Read the model definition and answer for the solid it produces. Units are mm, in the model's axes. A direction names the side the tool comes from. Coordinates: 2 decimals unless noted, no trailing zeros. Loops run counter-clockwise (first coordinate to the right, second up) from the corner with the lowest first, then second, coordinate; pieces in that order, holes last. Notation, with made-up numbers: M 18,-10.5 L 66,-10.5 A19 ccw 66,-0.5 Z; hole C -11.5,-0.5 d8. An arc over 180 degrees is marked long. One line per item, written item: value. Start each with the question number.
```python
from build123d import *

# Parameters (mm, degrees)
SKETCH1_W           = 20.5
SKETCH1_H           = 16.25
SKETCH1_R           = 1.625
BOSS_EXTRUDE1_DEPTH = 1.6
FILLET1_R           = 1
SKETCH2_W           = 2.5
SKETCH2_H           = 8
BOSS_EXTRUDE2_DEPTH = 2.5
FILLET2_R           = 0.5
SKETCH8_W           = 0.55
SKETCH8_H           = 0.55
SKETCH9_W           = 0.55
SKETCH9_H           = 0.55
SKETCH12_W          = 0.55
SKETCH12_H          = 0.55
SKETCH13_W          = 1.45
SKETCH13_H          = 1
CUT_EXTRUDE1_DEPTH  = 4


with BuildPart() as part:
    # Sketch1 → Boss-Extrude1 (new body)
    with BuildSketch(Plane(origin=(0, 0, 0), x_dir=(1, 0, 0), z_dir=(0, 1, 0))):
        Rectangle(SKETCH1_W, SKETCH1_H)
        with Locations(Location((7.625, 5.7, 0), (0, 0, 270))):
            Circle(SKETCH1_R, mode=Mode.SUBTRACT)
        with Locations(Location((7.625, -5.7, 0), (0, 0, 90))):
            Circle(SKETCH1_R, mode=Mode.SUBTRACT)
    extrude(amount=BOSS_EXTRUDE1_DEPTH)

    # Fillet1
    fillet1_edges = [part.edges().sort_by_distance(p)[0] for p in [
        (10.25, 0.8, 8.125),
        (-10.25, 0.8, 8.125),
        (-10.25, 0.8, -8.125),
        (10.25, 0.8, -8.125),
    ]]
    fillet(fillet1_edges, radius=FILLET1_R)

    # Sketch2 → Boss-Extrude2 (add)
    with BuildSketch(Plane(origin=(0, 1.6, 0), x_dir=(1, 0, 0), z_dir=(0, 1, 0))):
        with Locations((-9, 0)):
            Rectangle(SKETCH2_W, SKETCH2_H)
    extrude(amount=BOSS_EXTRUDE2_DEPTH)

    # Fillet2
    fillet2_edges = [part.edges().sort_by_distance(p)[0] for p in [
        (-7.75, 2.85, 4),
        (-7.75, 2.85, -4),
        (-10.25, 2.85, -4),
        (-10.25, 2.85, 4),
    ]]
    fillet(fillet2_edges, radius=FILLET2_R)

    # Sweep2: sweep along a path in Sketch5
    with BuildLine(Plane.XY.offset(-2.5)) as sweep2_path:
        Line((-9, 4.1), (-9, 4.85))
        ThreePointArc((-9, 4.85), (-8.682958383, 5.34027213), (-8.160059174, 5.6))
        Line((-8.160059174, 5.6), (-1, 5.6))
    # Sketch8 → Sweep2 (sweep)
    with BuildSketch(Plane(origin=(0, 4.1, 0), x_dir=(1, 0, 0), z_dir=(0, 1, 0))):
        with Locations((-9.001105099, 2.502876889)):
            Rectangle(SKETCH8_W, SKETCH8_H)
    sweep(path=sweep2_path.line, transition=Transition.RIGHT)

    # Sweep3: sweep along a path in Sketch6
    with BuildLine(Plane.XY.offset(2.5)) as sweep3_path:
        Line((-9, 4.1), (-9, 4.85))
        ThreePointArc((-9, 4.85), (-8.682958383, 5.34027213), (-8.160059174, 5.6))
        Line((-8.160059174, 5.6), (-1, 5.6))
    # Sketch9 → Sweep3 (sweep)
    with BuildSketch(Plane(origin=(0, 4.1, 0), x_dir=(1, 0, 0), z_dir=(0, 1, 0))):
        with Locations((-8.999962547, -2.498553748)):
            Rectangle(SKETCH9_W, SKETCH9_H)
    sweep(path=sweep3_path.line, transition=Transition.RIGHT)

    # Sweep4: sweep along a path in Sketch11
    with BuildLine(Plane.XY) as sweep4_path:
        Line((-9, 4.1), (-9, 4.85))
        ThreePointArc((-9, 4.85), (-8.682958383, 5.34027213), (-8.160059174, 5.6))
        Line((-8.160059174, 5.6), (-1, 5.6))
    # Sketch12 → Sweep4 (sweep)
    with BuildSketch(Plane(origin=(0, 4.1, 0), x_dir=(1, 0, 0), z_dir=(0, 1, 0))):
        with Locations((-9, 0)):
            Rectangle(SKETCH12_W, SKETCH12_H)
    sweep(path=sweep4_path.line, transition=Transition.RIGHT)

    # Sketch13 → Cut-Extrude1 (cut)
    with BuildSketch(Plane.XZ):
        with Locations((1.5, 4.755)):
            Rectangle(SKETCH13_W, SKETCH13_H)
    extrude(amount=-CUT_EXTRUDE1_DEPTH, mode=Mode.SUBTRACT)


solid = part.part
```
1) Consider line 1 along X through (y, z) = (1.15, 5.7); line 2 along Z through (x, y) = (1.25, 1.05) (3 decimals); line 3 along Z through (x, y) = (8, 1) (3 decimals). Determine where each line is inside the solid, lowest interval first.
2) Section A-A (z = 5.7) is taken. Determine the outline of the cut face in (x, y), then the cut area to 3 significant figures.
3) Section B-B (x = 7) is taken. Determine the outline of the cut face in (y, z) (3 decimals), then the cut area to 3 significant figures.
4) A tool of negligible diameter and unlimited length cuts with its end or side. For faces 1 (the face through (-6.1, 5.6, -2.228)), 2 (the face through (-7.75, 3, 0)), 3 (the face through (-9, 3, 4)), from which of +Z, -Z, +X, -X, +Y, -Y can it reach the whole face along a straight path? Write none if from no direction.
5) Flat-ended cylindrical pins translate along their axes: pin 1 (6 mm diameter, centred on x = -8, z = 2, fed in from -Y); pin 2 (1.4 mm diameter, centred on x = -5.5, y = 5, fed in from +Z); pin 3 (0.8 mm diameter, centred on x = -9, z = 2, fed in from +Y). Find the tip coordinate at first contact, or state that the pin passes through.
6) Section C-C (x = -2) is taken. Determine the outline of the cut face in (y, z) (3 decimals), then the cut area to 3 significant figures.
7) Section D-D (y = 3.6) is taken. Determine the outline of the cut face in (x, z), then the cut area to 3 significant figures.
8) For a pull along Z with two mould halves and no side action, classify faces 4 (the face through (0, 0, 0)), 5 (the face through (1, 1, 4.255)), 6 (the face through (-6, 5.6, -2.778)) as released by +Z, released by -Z, zero draft, split by the parting line, or undercut.
Results found:
1. line 1: x = -10.25 to 6, 9.25 to 10.25
1. line 2: z = -8.125 to 4.255, 5.255 to 8.125
1. line 3: z = -8.125 to -7.281, -4.119 to 4.119, 7.281 to 8.125
2. outline: M -10.25,0 L 6,0 L 6,1.6 L -10.25,1.6 Z; M 9.25,0 L 10.25,0 L 10.25,1.6 L 9.25,1.6 Z
2. area: 27.6 mm²
3. outline: M 0,-8.125 L 1.6,-8.125 L 1.6,-7.2 L 0,-7.2 Z; M 0,-4.2 L 1.6,-4.2 L 1.6,4.2 L 0,4.2 Z; M 0,7.2 L 1.6,7.2 L 1.6,8.125 L 0,8.125 Z
3. area: 16.4 mm²
4. face 1: +X, -X, +Y
4. face 2: +Z, -Z, +X
4. face 3: +Z, +X, -X, +Y
5. pin 1: stops at y = 0
5. pin 2: stops at z = 2.77
5. pin 3: stops at y = 5.69
6. outline: M 0,-8.125 L 1.6,-8.125 L 1.6,8.125 L 0,8.125 Z; M 5.325,-0.275 L 5.875,-0.275 L 5.875,0.275 L 5.325,0.275 Z; M 5.325,2.224 L 5.875,2.224 L 5.875,2.774 L 5.325,2.774 Z; M 5.326,-2.778 L 5.876,-2.778 L 5.876,-2.228 L 5.326,-2.228 Z
6. area: 26.9 mm²
7. outline: M -10.25,-3.5 A0.5 ccw -9.75,-4 L -8.25,-4 A0.5 ccw -7.75,-3.5 L -7.75,3.5 A0.5 ccw -8.25,4 L -9.75,4 A0.5 ccw -10.25,3.5 Z
7. area: 19.8 mm²
8. face 4: zero draft
8. face 5: undercut
8. face 6: released by -Z
